from build123d import *

# Parameters (mm, degrees)
EXTRUDE_1_DEPTH     = 15
CUT_EXTRUDE_START   = -15
CUT_EXTRUDE_1_DEPTH = 15
SKETCH_7_R          = 10.1
CUT_EXTRUDE_2_DEPTH = 2


with BuildPart() as part:
    # ｽｹｯﾁ4 → ﾎﾞｽ - 押し出し1 (new body)
    with BuildSketch(Plane.XY):
        with BuildLine():
            Line((-53.623111018, -124.995132678), (-58.940636287, -129.45706617))
            ThreePointArc((-58.940636287, -129.45706617), (-60.005384698, -131.552012131), (-59.233530865, -133.771635843))
            ThreePointArc((-59.233530865, -133.771635843), (57.362306223, -135.763481103), (52.076178918, -19.270504783))
            Line((52.076178918, -19.270504783), (10.606601718, 10.606601718))
            ThreePointArc((10.606601718, 10.606601718), (-10.606601718, 10.606601718), (-10.606601718, -10.606601718))
            Line((-10.606601718, -10.606601718), (14.536280154, -62.889638219))
            ThreePointArc((14.536280154, -62.889638219), (14.918089499, -66.109676181), (13.244185189, -68.886809092))
            Line((13.244185189, -68.886809092), (-53.623111018, -124.995132678))
        make_face()
        with BuildLine():
            Line((21.232400696, -76.813798404), (45.844843506, -127.993820346))
            ThreePointArc((45.844843506, -127.993820346), (46.221944165, -131.235480845), (44.518718993, -134.019289696))
            ThreePointArc((44.518718993, -134.019289696), (-2.231208213, -149.964431749), (-47.870174388, -131.072951785))
            ThreePointArc((-47.870174388, -131.072951785), (-48.817477846, -128.802229421), (-47.747678417, -126.586582094))
            Line((-47.747678417, -126.586582094), (13.511229465, -75.151532228))
            ThreePointArc((13.511229465, -75.151532228), (17.77869109, -74.092739753), (21.232400696, -76.813798404))
        make_face(mode=Mode.SUBTRACT)
    extrude(amount=EXTRUDE_1_DEPTH)

    # ｽｹｯﾁ6 → ｶｯﾄ - 押し出し1 (cut)
    with BuildSketch(Plane.XY.offset(15).offset(CUT_EXTRUDE_START)):
        with BuildLine():
            Line((49.189589797, -118.797265215), (2.201751786, -21.089020696))
            ThreePointArc((2.201751786, -21.089020696), (1.989274209, -17.268089629), (4.540836142, -14.416039025))
            Line((4.540836142, -14.416039025), (6.483415605, -13.48185369))
            Line((6.483415605, -13.48185369), (10.219658847, -11.685096486))
            ThreePointArc((10.219658847, -11.685096486), (11.747077013, -11.232198087), (13.339423466, -11.282754846))
            ThreePointArc((13.339423466, -11.282754846), (64.738421392, -53.37413296), (57.826055334, -119.448033215))
            ThreePointArc((57.826055334, -119.448033215), (53.319931874, -121.616182211), (49.189589797, -118.797265215))
        make_face()
    extrude(amount=CUT_EXTRUDE_1_DEPTH, mode=Mode.SUBTRACT)

    # ｽｹｯﾁ7 → ｶｯﾄ - 押し出し2 (cut)
    with BuildSketch(Plane.XY.offset(15)):
        Circle(SKETCH_7_R)
    extrude(amount=-CUT_EXTRUDE_2_DEPTH, mode=Mode.SUBTRACT)


solid = part.part
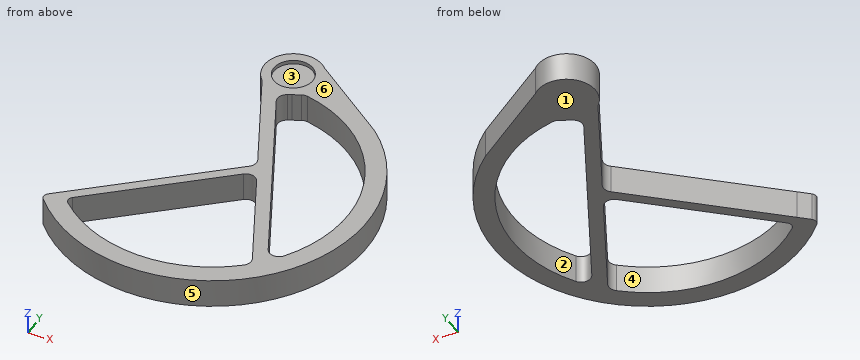
Geometry check sheet. Reference: the model listing, model coordinates, mm. Face numbers are marked on the shaded views. A direction names the side the tool comes from. Give positions to 0.01 mm unless a question says otherwise; leave off trailing zeros. Write each loop counter-clockwise with the first axis right and the second up, starting at its lowest first coordinate (ties: lowest second). Pieces come first, ordered by that corner, then holes. Notation, with made-up numbers: M 14,31.25 L 29,31.25 A12 ccw 29,39.25 Z; hole C -38.5,55.5 d7. An arc over 180 degrees is marked long. Answer as CSV lines item,"result". Start each with the question number.
Q1. Section check B-B, the plane y = -112. Record the cut outline in (x, z), then the cut area to 3 significant figures.
Q2. Section check C-C, the plane x = -41.5. Record the cut outline in (y, z), then the cut area to 3 significant figures.
Q3. Release check for a two-part mould opening along X. For the marked faces 4, 5 and 6 record: pulls with the +X half, pulls with the -X half, needs draft (parallel to the pull), parting line crosses it, or undercut.
Q4. Section check D-D, the plane y = 0. Record the cut outline in (x, z), then the cut area to 3 significant figures.
Q5. Go/stop test with flat-tipped pins: pin 1 (1.5 mm diameter, centred on x = -25, z = 6.5, fed in from -Y); pin 2 (1.5 mm diameter, centred on x = 56, z = 8.5, fed in from -Y); pin 3 (1.5 mm diameter, centred on y = -122.5, z = 2, fed in from -X). Record where each tip stops, or that it passes through.
Q6. Tool access check on the marked faces 1, 2 and 3. Record the directions out of +Z, -Z, +X, -X, +Y, -Y that give a thin tool (end or side, any length) a straight path to the whole face; none if there is none.
Q7. Material ranges on L1, parallel to Y at x = 0, z = 14.1; L2, parallel to Y at x = 7, z = 5; L3, parallel to X at y = -86, z = 6, recorded low to high.
Q8. Section check A-A, the plane z = 7. Record the cut outline in (x, y), then the cut area to 3 significant figures.
Geometry says:
1,outline,"M -38.14,0 L -30.38,0 L -30.38,15 L -38.14,15 Z; M 38.15,0 L 45.92,0 L 45.92,15 L 38.15,15 Z; M 62.26,0 L 73.32,0 L 73.32,15 L 62.26,15 Z"
1,area,"399 mm^2"
2,outline,"M -148.39,0 L -136.37,0 L -136.37,15 L -148.39,15 Z; M -121.34,0 L -114.82,0 L -114.82,15 L -121.34,15 Z"
2,area,"278 mm^2"
3,face 4,"undercut"
3,face 5,"parting line crosses it"
3,face 6,"needs draft"
4,outline,"M -15,0 L 25.33,0 L 25.33,15 L 10.1,15 L 10.1,13 L -10.1,13 L -10.1,15 L -15,15 Z"
4,area,"565 mm^2"
5,pin 1,"y = -156.24"
5,pin 2,"y = -137.86"
5,pin 3,"x = -51.54"
6,face 1,"-Z, +X, -X, +Y, -Y"
6,face 2,"+Z, -Z"
6,face 3,"+Z"
7,L1,"-160 to -150, -86.5 to -80, -32.66 to -10.1, 10.1 to 15"
7,L2,"-159.69 to -149.65, -80.62 to -74.13, -47.22 to -31.07, -13.23 to 13.27"
7,L3,"-7.15 to 0.59, 25.65 to 33.42, 69.74 to 79.77"
8,outline,"M -59.23,-133.77 A80 ccw long 52.08,-19.27 L 10.61,10.61 A15 ccw -10.61,-10.61 L 14.54,-62.89 A5 cw 13.24,-68.89 L -58.94,-129.46 A3 ccw Z; hole M -47.87,-131.07 A70 ccw 44.52,-134.02 A5 ccw 45.84,-127.99 L 21.23,-76.81 A5 ccw 13.51,-75.15 L -47.75,-126.59 A3 ccw Z; hole M 2.2,-21.09 L 49.19,-118.8 A5 ccw 57.83,-119.45 A70 ccw 13.34,-11.28 A5 ccw 10.22,-11.69 L 4.54,-14.42 A5 ccw Z"
8,area,"5,070 mm^2"
